Design review of the part built by this model. Coordinates are the model's own, in mm. A direction names the side the tool comes from. Coordinates: 2 decimals unless noted, no trailing zeros. Write each loop counter-clockwise with the first axis right and the second up, starting at its lowest first coordinate (ties: lowest second). Pieces come first, ordered by that corner, then holes.
Q1. The part is to be moulded in two halves that separate along X. For faces 3 (the face through (-256.168, -360, -15)), 4 (the face through (-499.06, -59.06, -15.07)), 5 (the face through (-271, -508.604, -15)), say which applies: +X half, -X half, draft (parallel to the pull), parting line (faces both ways), or undercut.
Q2. Machinability: for faces 1 (the face through (-427, -393.104, -15)), 2 (the face through (-562.85, -490.73, -14.93)), which of the approach directions +Z, -Z, +X, -X, +Y, -Y give a long, thin tool a straight path to every point of the face, cutting with its end or side? Answer none if there is none.
Q3. Clearance check with flat-ended pins moving along their axes: pin 1 Ø3 at (x, z) = (-391.5, -13) entering from -Y; pin 2 Ø3 at (y, z) = (-354.5, -18) entering from -X. State where each tip first meets the part, or that it passes through.
Q4. To check wall thickness, follow probe 1 along X at (y, z) = (-425.5, -12.25); probe 2 along Y at (x, z) = (-447, -15.5); probe 3 along X at (y, z) = (-184, -12.5). State the ranges of each line that lie inside material, in increasing order.
Q5. Add section C-C, the plane y = -261.5. Give the boundary of the cut face in (x, z).
Q6. Add section A-A, the plane x = -438.5. Give the boundary of the cut face in (y, z), plus the area to 4 significant figures.
Q7. Add section B-B, the plane y = -115.5. Give the boundary of the cut face in (x, z).
Q8. Add section D-D, the plane z = -17. Give the number of separate pieces and of enclosed holes in the cut face, plus the area to 3 significant figures.
from build123d import *

# Parameters (mm, degrees)
SZKIC1_W                    = 358
SZKIC1_H                    = 451.5
DODANIE_WYCI_GNI_CIE1_DEPTH = 10
WYTNIJ_WYCI_GNI_CIE1_DEPTH  = 10
WYTNIJ_WYCI_GNI_CIE2_DEPTH  = 10
WYTNIJ_WYCI_GNI_CIE3_DEPTH  = 10
SZKIC8_W                    = 6.4
SZKIC8_H                    = 20.4
WYTNIJ_WYCI_GNI_CIE4_DEPTH  = 10
SZYK_LINIOWY1_COUNT         = 6
SZYK_LINIOWY1_PITCH         = 60
SZKIC9_R                    = 1.55
WYTNIJ_WYCI_GNI_CIE5_DEPTH  = 10
SZYK_LINIOWY2_COUNT         = 4
SZYK_LINIOWY2_PITCH         = 120
SZKIC12_W                   = 12.4
SZKIC12_H                   = 32.68
WYTNIJ_WYCI_GNI_CIE7_DEPTH  = 10
SZKIC13_R                   = 1.55
WYTNIJ_WYCI_GNI_CIE8_DEPTH  = 10
SZKIC15_R                   = 1.5
WYTNIJ_WYCI_GNI_CIE9_DEPTH  = 10
SZKIC17_R                   = 1.55
WYTNIJ_WYCI_GNI_CIE10_DEPTH = 10
SZKIC19_W                   = 20.4
SZKIC19_H                   = 6.4
SZKIC19_W_2                 = 30.4
WYTNIJ_WYCI_GNI_CIE11_DEPTH = 10
SZKIC23_R                   = 1.55
SZKIC23_W                   = 15.4
SZKIC23_H                   = 6.4
SZKIC23_W_2                 = 17.9
WYTNIJ_WYCI_GNI_CIE12_DEPTH = 10
WYTNIJ_WYCI_GNI_CIE14_DEPTH = 10
SZKIC32_R                   = 1.55
SZKIC32_W                   = 10.4
SZKIC32_H                   = 6.4
SZKIC32_W_2                 = 15.4
WYTNIJ_WYCI_GNI_CIE15_DEPTH = 10
WYTNIJ_WYCI_GNI_CIE16_DEPTH = 10
SZYK_LINIOWY3_COUNT         = 2
SZYK_LINIOWY3_PITCH         = 155
WYTNIJ_WYCI_GNI_CIE17_DEPTH = 10


with BuildPart() as part:
    # Szkic1 → Dodanie-wyciągnięcie1 (new body)
    with BuildSketch(Plane.XY.offset(-20)):
        with Locations((-429.368459045, -282.853962956)):
            Rectangle(SZKIC1_W, SZKIC1_H)
    extrude(amount=DODANIE_WYCI_GNI_CIE1_DEPTH)

    # Szkic2 → Wytnij-wyciągnięcie1 (cut)
    with BuildSketch(Plane(origin=(0, 0, -20), x_dir=(-1, 0, 0), z_dir=(0, 0, -1))):
        with BuildLine():
            Line((608.368459045, -387.603962956), (502.621218356, -63.997823625))
            ThreePointArc((502.621218356, -63.997823625), (498.986913201, -59.008859704), (493.115856793, -57.103962956))
            Line((493.115856793, -57.103962956), (500.368459045, -57.103962956))
            Line((500.368459045, -57.103962956), (608.368459045, -57.103962956))
            Line((608.368459045, -57.103962956), (608.368459045, -387.603962956))
        make_face()
    extrude(amount=-WYTNIJ_WYCI_GNI_CIE1_DEPTH, mode=Mode.SUBTRACT)

    # Szkic3 → Wytnij-wyciągnięcie2 (cut)
    with BuildSketch(Plane.XY.offset(-10)):
        with BuildLine():
            Line((-570.368459045, -508.603962956), (-290.368459045, -508.603962956))
            ThreePointArc((-290.368459045, -508.603962956), (-297.690789516, -490.926293426), (-315.368459045, -483.603962956))
            Line((-315.368459045, -483.603962956), (-545.368459045, -483.603962956))
            ThreePointArc((-545.368459045, -483.603962956), (-563.046128575, -490.926293426), (-570.368459045, -508.603962956))
        make_face()
    extrude(amount=-WYTNIJ_WYCI_GNI_CIE2_DEPTH, mode=Mode.SUBTRACT)

    # Szkic4 → Wytnij-wyciągnięcie3 (cut)
    with BuildSketch(Plane.XY.offset(-10)):
        with BuildLine():
            Line((-491.890848015, -393.103962956), (-360.368459045, -393.103962956))
            ThreePointArc((-360.368459045, -393.103962956), (-332.084187798, -381.388234203), (-320.368459045, -353.103962956))
            Line((-320.368459045, -353.103962956), (-320.368459045, -217.103962956))
            ThreePointArc((-320.368459045, -217.103962956), (-332.084187798, -188.819691708), (-360.368459045, -177.103962956))
            Line((-360.368459045, -177.103962956), (-447.449093098, -177.103962956))
            ThreePointArc((-447.449093098, -177.103962956), (-470.93331873, -184.723549949), (-485.470539353, -204.679405632))
            Line((-485.470539353, -204.679405632), (-529.91229427, -340.679405632))
            ThreePointArc((-529.91229427, -340.679405632), (-524.271261022, -376.588188587), (-491.890848015, -393.103962956))
        make_face()
    extrude(amount=-WYTNIJ_WYCI_GNI_CIE3_DEPTH, mode=Mode.SUBTRACT)

    # Szkic8 → Wytnij-wyciągnięcie4 (cut)
    with BuildSketch(Plane.XY.offset(-10)):
        with Locations((-259.368459045, -119.603962956)):
            Rectangle(SZKIC8_W, SZKIC8_H)
    wytnij_wyci_gni_cie4 = extrude(amount=-WYTNIJ_WYCI_GNI_CIE4_DEPTH, mode=Mode.SUBTRACT)

    # Szyk liniowy1: Wytnij-wyciągnięcie4 ×6
    with Locations(*[(0, -i * SZYK_LINIOWY1_PITCH, 0) for i in range(1, SZYK_LINIOWY1_COUNT)]):
        add(wytnij_wyci_gni_cie4, mode=Mode.SUBTRACT)

    # Szkic9 → Wytnij-wyciągnięcie5 (cut)
    with BuildSketch(Plane.XY.offset(-10)):
        with Locations((-259.368459045, -89.603962956)):
            Circle(SZKIC9_R)
    wytnij_wyci_gni_cie5 = extrude(amount=-WYTNIJ_WYCI_GNI_CIE5_DEPTH, mode=Mode.SUBTRACT)

    # Szyk liniowy2: Wytnij-wyciągnięcie5 ×4
    with Locations(*[(0, -i * SZYK_LINIOWY2_PITCH, 0) for i in range(1, SZYK_LINIOWY2_COUNT)]):
        add(wytnij_wyci_gni_cie5, mode=Mode.SUBTRACT)

    # Szkic12 → Wytnij-wyciągnięcie7 (cut)
    with BuildSketch(Plane.XY.offset(-10)):
        with Locations((-596.368459045, -422.463962956)):
            Rectangle(SZKIC12_W, SZKIC12_H)
    extrude(amount=-WYTNIJ_WYCI_GNI_CIE7_DEPTH, mode=Mode.SUBTRACT)

    # Szkic13 → Wytnij-wyciągnięcie8 (cut)
    with BuildSketch(Plane.XY.offset(-10)):
        with Locations((-593.368459045, -397.873962956)):
            Circle(SZKIC13_R)
        with Locations((-593.368459045, -446.553962956)):
            Circle(SZKIC13_R)
    extrude(amount=-WYTNIJ_WYCI_GNI_CIE8_DEPTH, mode=Mode.SUBTRACT)

    # Szkic15 → Wytnij-wyciągnięcie9 (cut)
    with BuildSketch(Plane.XY.offset(-10)):
        with Locations((-295.368459045, -471.603962956)):
            Circle(SZKIC15_R)
        with Locations((-323.368459045, -471.603962956)):
            Circle(SZKIC15_R)
        with Locations((-375.368459045, -471.603962956)):
            Circle(SZKIC15_R)
        with Locations((-427.368459045, -471.603962956)):
            Circle(SZKIC15_R)
        with Locations((-531.368459045, -471.603962956)):
            Circle(SZKIC15_R)
        with Locations((-479.368459045, -471.603962956)):
            Circle(SZKIC15_R)
        with Locations((-583.368459045, -471.603962956)):
            Circle(SZKIC15_R)
        with Locations((-338.368459045, -449.412668339)):
            Circle(SZKIC15_R)
    extrude(amount=-WYTNIJ_WYCI_GNI_CIE9_DEPTH, mode=Mode.SUBTRACT)

    # Szkic17 → Wytnij-wyciągnięcie10 (cut)
    with BuildSketch(Plane.XY.offset(-10)):
        with Locations((-455.868459045, -137.814883619)):
            Circle(SZKIC17_R)
        with Locations((-455.868459045, -82.814883619)):
            Circle(SZKIC17_R)
        with Locations((-465.868459045, -137.814883619)):
            Circle(SZKIC17_R)
        with Locations((-465.868459045, -82.814883619)):
            Circle(SZKIC17_R)
        Polygon((-471.068459045, -125.803962956), (-460.868459045, -125.803962956), (-450.668459045, -125.803962956), (-450.668459045, -95.403962956), (-460.868459045, -95.403962956), (-471.068459045, -95.403962956), align=None)
    wytnij_wyci_gni_cie10 = extrude(amount=-WYTNIJ_WYCI_GNI_CIE10_DEPTH, mode=Mode.SUBTRACT)

    # Szkic19 → Wytnij-wyciągnięcie11 (cut)
    with BuildSketch(Plane.XY.offset(-10)):
        with Locations((-480.368459045, -66.103962956)):
            Rectangle(SZKIC19_W, SZKIC19_H)
        with Locations((-393.118459045, -66.103962956)):
            Rectangle(SZKIC19_W_2, SZKIC19_H)
        with Locations((-305.868459045, -66.103962956)):
            Rectangle(SZKIC19_W, SZKIC19_H)
    extrude(amount=-WYTNIJ_WYCI_GNI_CIE11_DEPTH, mode=Mode.SUBTRACT)

    # Szkic23 → Wytnij-wyciągnięcie12 (cut)
    with BuildSketch(Plane.XY.offset(-10)):
        with Locations((-322.868459045, -420.103962956)):
            Circle(SZKIC23_R)
        with Locations((-278.868459045, -420.103962956)):
            Rectangle(SZKIC23_W, SZKIC23_H)
        with Locations((-310.118459045, -420.103962956)):
            Rectangle(SZKIC23_W_2, SZKIC23_H)
    extrude(amount=-WYTNIJ_WYCI_GNI_CIE12_DEPTH, mode=Mode.SUBTRACT)

    # Szkic29 → Wytnij-wyciągnięcie14 (cut)
    with BuildSketch(Plane.XY.offset(-10)):
        Polygon((-323.403118877, -381.907994616), (-322.29177054, -388.210764235), (-310.89994388, -386.202077835), (-312.011292217, -379.899308216), align=None)
        Polygon((-281.383771099, -374.498849891), (-280.272422762, -380.80161951), (-266.091191118, -378.301085752), (-267.202539455, -371.998316132), align=None)
    extrude(amount=-WYTNIJ_WYCI_GNI_CIE14_DEPTH, mode=Mode.SUBTRACT)

    # Szkic32 → Wytnij-wyciągnięcie15 (cut)
    with BuildSketch(Plane.XY.offset(-10)):
        with Locations((-307.650240695, -400.103962956)):
            Circle(SZKIC32_R)
        with Locations((-322.368459045, -400.103962956)):
            Rectangle(SZKIC32_W, SZKIC32_H)
        with Locations((-274.868459045, -400.103962956)):
            Rectangle(SZKIC32_W_2, SZKIC32_H)
    extrude(amount=-WYTNIJ_WYCI_GNI_CIE15_DEPTH, mode=Mode.SUBTRACT)

    # Szkic34 → Wytnij-wyciągnięcie16 (cut)
    with BuildSketch(Plane(origin=(0, 0, -20), x_dir=(-1, 0, 0), z_dir=(0, 0, -1))):
        with BuildLine():
            Line((607.281290895, -383.676301549), (608.368459045, -387.603962956))
            Line((608.368459045, -387.603962956), (608.368459045, -391.679310636))
            ThreePointArc((608.368459045, -391.679310636), (608.095424544, -387.641053306), (607.281290895, -383.676301549))
        make_face()
    extrude(amount=-WYTNIJ_WYCI_GNI_CIE16_DEPTH, mode=Mode.SUBTRACT)

    # Szyk liniowy3: Wytnij-wyciągnięcie10 ×2
    with Locations(*[(i * SZYK_LINIOWY3_PITCH, 0, 0) for i in range(1, SZYK_LINIOWY3_COUNT)]):
        add(wytnij_wyci_gni_cie10, mode=Mode.SUBTRACT)

    # Szkic35 → Wytnij-wyciągnięcie17 (cut)
    with BuildSketch(Plane.XY.offset(-10)):
        with BuildLine():
            Line((-260.368459045, -57.103962956), (-250.368459045, -57.103962956))
            Line((-250.368459045, -57.103962956), (-250.368459045, -67.103962956))
            ThreePointArc((-250.368459045, -67.103962956), (-253.297391233, -60.032895144), (-260.368459045, -57.103962956))
        make_face()
    extrude(amount=-WYTNIJ_WYCI_GNI_CIE17_DEPTH, mode=Mode.SUBTRACT)


solid = part.part
Here are the results:
1. face 3: undercut
1. face 4: -X half
1. face 5: draft
2. face 1: +Z, -Z
2. face 2: +Z, -Z, -Y
3. pin 1: stops at y = -483.6
3. pin 2: stops at x = -598.04
4. probe 1: x = -608.37 to -602.57, -590.17 to -262.57, -256.17 to -250.37
4. probe 2: y = -483.6 to -393.1, -177.1 to -57.1
4. probe 3: x = -541.84 to -469.9, -337.92 to -262.57, -256.17 to -250.37
5. outline: (-567.16, -20) - (-504.04, -20) - (-504.04, -10) - (-567.16, -10) - close; (-320.37, -20) - (-250.37, -20) - (-250.37, -10) - (-320.37, -10) - close
6. outline: (-483.6, -20) - (-393.1, -20) - (-393.1, -10) - (-483.6, -10) - close; (-177.1, -20) - (-57.1, -20) - (-57.1, -10) - (-177.1, -10) - close
6. area: 2,105 mm2
7. outline: (-519.45, -20) - (-471.07, -20) - (-471.07, -10) - (-519.45, -10) - close; (-450.67, -20) - (-316.07, -20) - (-316.07, -10) - (-450.67, -10) - close; (-295.67, -20) - (-262.57, -20) - (-262.57, -10) - (-295.67, -10) - close; (-256.17, -20) - (-250.37, -20) - (-250.37, -10) - (-256.17, -10) - close
8. separate pieces: 1
8. enclosed holes: 43
8. area: 93,600 mm2
